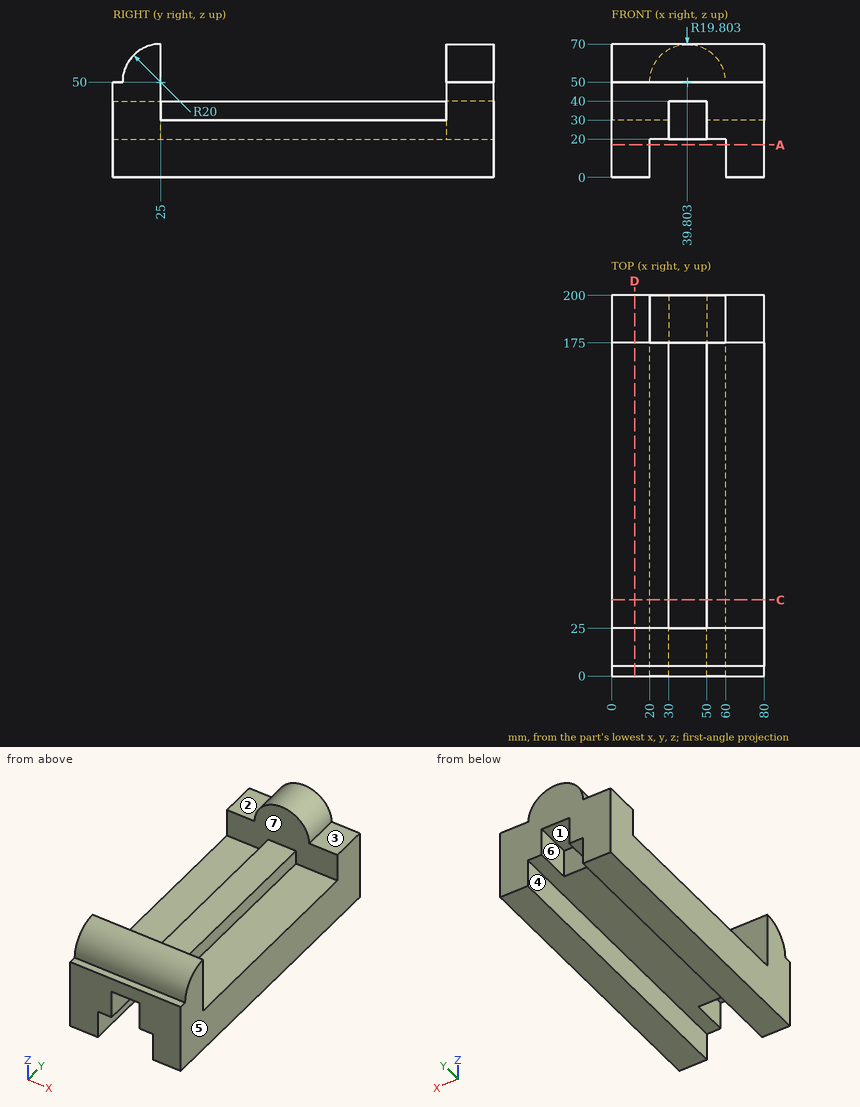
Input: dimensioned drawing with shaded views. Units: mm. Origin: part minimum x, y, z. A direction names the side the tool comes from. Coordinates: 2 decimals unless noted, no trailing zeros. Loops run counter-clockwise (first coordinate to the right, second up) from the corner with the lowest first, then second, coordinate; pieces in that order, holes last.
Q1. Section C-C, the plane y = 40. Return the cut outline in (x, z), and give its area (3 significant figures).
Results are:
outline: (0, 0) - (20, 0) - (20, 20) - (60, 20) - (60, 0) - (80, 0) - (80, 30) - (50, 30) - (50, 40) - (30, 40) - (30, 30) - (0, 30) - close
area: 1,800 mm2
Q2. Section A-A, the plane z = 17. Return the cut outline in (x, y), and give its area (3 significant figures).
Results are:
outline: (0, 0) - (20, 0) - (20, 200) - (0, 200) - close; (60, 0) - (80, 0) - (80, 200) - (60, 200) - close
area: 8,000 mm2
Q3. Mould query, pull axis X, two halves, no side actions, for the marked faces 4, 5, 6 and 7. Classes: +X half, -X half, draft (parallel to the pull), parting line (faces both ways), or undercut.
Results are:
face 4: undercut
face 5: +X half
face 6: undercut
face 7: draft
Q4. Line query: line 1 along Y through (x, z) = (65.5, 39.5); line 2 along X through (y, z) = (45, 4); line 3 along X through (y, z) = (183.5, 31). Output: solid intervals per line, ascending.
Results are:
line 1: y = 0 to 25, 175 to 200
line 2: x = 0 to 20, 60 to 80
line 3: x = 0 to 30, 50 to 80
Q5. Section D-D, the plane x = 12. Return the cut outline in (y, z), and give its area (3 significant figures).
Results are:
outline: (0, 0) - (200, 0) - (200, 50) - (175, 50) - (175, 30) - (25, 30) - (25, 70) arc R20 ccw to (5, 50) - (0, 50) - close
area: 7,310 mm2
Q6. Contact query for flat-ended pins moving along their axis: pin 1 (10 mm diameter, centred on x = 39, y = 171.5, fed in from +Z); pin 2 (5 mm diameter, centred on x = 53.5, y = 158, fed in from -Z); pin 3 (6 mm diameter, centred on x = 68, y = 189.5, fed in from +Z). Output: stop coordinate, or through.
Results are:
pin 1: stops at z = 69.8
pin 2: stops at z = 20
pin 3: stops at z = 50
Q7. Set-up query: the marked faces 1, 2 and 3. Return all of +Z, -Z, +X, -X, +Y, -Y with unobstructed straight access to the full face (end or side cutting, diameter ignored); none if empty.
Results are:
face 1: -Z, +Y
face 2: +Z, -X, +Y
face 3: +Z, +X, +Y
